```python
from build123d import *

# Parameters (mm, degrees)
F0_W     = 635
F0_H     = 1016
F1_DEPTH = 635
F2_SIZE  = 139.7
F3_T     = -2.54


with BuildPart() as f1:
    # F0 (on Front) → F1 (new body)
    with BuildSketch(Plane.XZ):
        with Locations((-2.180368, 82.699301)):
            Rectangle(F0_W, F0_H)
    extrude(amount=F1_DEPTH)

    # F2
    f2_edges = [f1.edges().sort_by_distance(p)[0] for p in [
        (315.319632, -317.5, 590.699301),
        (-2.180368, -635, 590.699301),
        (-319.680368, -317.5, 590.699301),
        (-2.180368, 0, 590.699301),
        (315.319632, -635, 82.699301),
        (315.319632, 0, 82.699301),
        (-319.680368, -635, 82.699301),
        (-2.180368, -635, -425.300699),
        (315.319632, -317.5, -425.300699),
        (-319.680368, 0, 82.699301),
        (-319.680368, -317.5, -425.300699),
        (-2.180368, 0, -425.300699),
    ]]
    chamfer(f2_edges, length=F2_SIZE)

    # F3
    f3_openings = [f1.faces().sort_by_distance(p)[0] for p in [
        (-319.680368, -317.5, 82.699301),
    ]]
    offset(amount=F3_T, openings=f3_openings)


solid = f1.part
```
Geometry: final body of the model. Coordinates: model frame, mm. A direction names the side the tool comes from. Round coordinates to 2 decimals unless told otherwise and drop trailing zeros. Write each loop counter-clockwise with the first axis right and the second up, starting at its lowest first coordinate (ties: lowest second). Pieces come first, ordered by that corner, then holes. Notation, with made-up numbers: (-10, 23.25) -> (27, 23.25) arc R22 cw to (27, 45.25) -> close; hole circle Ø4 at (20.5, 20.25). An arc over 180 degrees is marked (long way). Use CSV: the item, a comma, the result in double quotes. Start each with the question number.
Q1. Section C-C (z = 27). Return loops of the section in (x, y), plus the area to 3 significant figures.
Q2. Section B-B (x = -120). Return loops of the section in (y, z), plus the area to 3 significant figures.
Q3. Section A-A (y = -301.5). Return loops of the section in (x, z), plus the area to 3 significant figures.
Q4. Section D-D (z = 490). Return loops of the section in (x, y).
Q5. Line query: L1, parallel to Z at x = -29.5, y = -155; L2, parallel to Y at x = -150, z = -118; L3, parallel to X at y = -113.5, z = -129.5. Output: solid intervals per line, ascending.
Q6. Pull-direction query (X, two-part tool) for faces 3 (the face through (-5, -566, 520)), 4 (the face through (-248.85, -315.01, -356.43)), 5 (the face through (-248.32, -315.02, 518.77)); classes: pulls with the +X half, pulls with the -X half, needs draft (parallel to the pull), parting line crosses it, or undercut.
Q7. Reachability of faces 1 (the face through (-248.32, -71.93, 77.55)), 2 (the face through (244.49, -68.87, 77.54)) from +Z, -Z, +X, -X, +Y, -Y: full face, straight path, thin tool, end or side. Return the list, or none.
Q8. First-contact query: pin 1 Ø4 at (y, z) = (-383, -177) entering from -X; pin 2 Ø8 at (x, y) = (-252.5, -327) entering from -Z; pin 3 Ø10 at (x, y) = (-236.5, -251) entering from +Z. Flat tips, straight axial feed; report the tip coordinate or a pass-through.
Result sheet:
1,outline,"(-319.68, -495.3) -> (-179.98, -635) -> (175.62, -635) -> (315.32, -495.3) -> (315.32, -139.7) -> (175.62, 0) -> (-179.98, 0) -> (-319.68, -139.7) -> (-319.68, -143.29) -> (-178.93, -2.54) -> (174.57, -2.54) -> (312.78, -140.75) -> (312.78, -494.25) -> (174.57, -632.46) -> (-178.93, -632.46) -> (-319.68, -491.71) -> close"
1,area,"4,710 mm²"
2,outline,"(-635, -285.6) -> (-495.3, -425.3) -> (-139.7, -425.3) -> (0, -285.6) -> (0, 451) -> (-139.7, 590.7) -> (-495.3, 590.7) -> (-635, 451) -> close; hole (-632.46, -284.55) -> (-494.25, -422.76) -> (-140.75, -422.76) -> (-2.54, -284.55) -> (-2.54, 449.95) -> (-140.75, 588.16) -> (-494.25, 588.16) -> (-632.46, 449.95) -> close"
2,area,"7,530 mm²"
3,outline,"(-319.68, -285.6) -> (-179.98, -425.3) -> (175.62, -425.3) -> (315.32, -285.6) -> (315.32, 451) -> (175.62, 590.7) -> (-179.98, 590.7) -> (-319.68, 451) -> (-319.68, 447.41) -> (-178.93, 588.16) -> (174.57, 588.16) -> (312.78, 449.95) -> (312.78, -284.55) -> (174.57, -422.76) -> (-178.93, -422.76) -> (-319.68, -282.01) -> close"
3,area,"5,680 mm²"
4,outline,"(-280.68, -495.3) -> (-179.98, -596) -> (175.62, -596) -> (276.32, -495.3) -> (276.32, -139.7) -> (175.62, -39) -> (-179.98, -39) -> (-280.68, -139.7) -> close; hole (-277.09, -494.49) -> (-179.17, -592.41) -> (174.81, -592.41) -> (272.73, -494.49) -> (272.73, -140.51) -> (174.81, -42.59) -> (-179.17, -42.59) -> (-277.09, -140.51) -> close"
5,L1,"-425.3 to -422.76, 588.16 to 590.7"
5,L2,"-635 to -632.46, -2.54 to 0"
5,L3,"-293.48 to -289.89, 285.53 to 289.12"
6,face 3,"needs draft"
6,face 4,"pulls with the -X half"
6,face 5,"undercut"
7,face 1,"none"
7,face 2,"+Z, -Z, +X, +Y"
8,pin 1,"x = 312.78"
8,pin 2,"z = -356.78"
8,pin 3,"z = 539.18"
